Print and shaded views of the part. All mm, measured from the part's lowest x, y and z. Give positions to 0.01 mm unless a question says otherwise; leave off trailing zeros. Loops run counter-clockwise (first coordinate to the right, second up) from the corner with the lowest first, then second, coordinate; pieces in that order, holes last. Notation, with made-up numbers: M 3.25,4.5 L 55.25,4.5 A14 cw 55.25,10.5 Z; hole C 70,4 d10. An arc over 180 degrees is marked long. Answer in a Markdown table with one row per item.
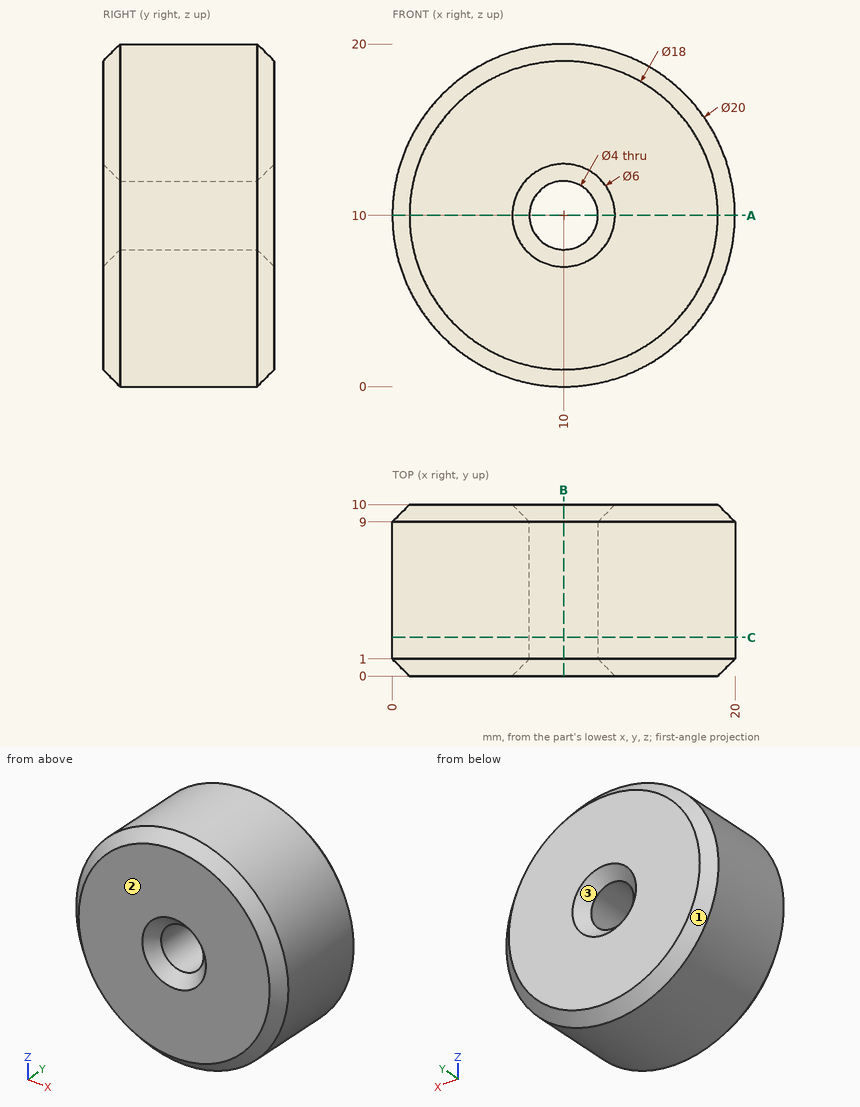
(1) Saw through at A-A, the plane z = 10. Give the cut face in (x, y).
Established:
| item | result |
|---|---|
| outline | M 0,1 L 1,0 L 7,0 L 8,1 L 8,9 L 7,10 L 1,10 L 0,9 Z; M 12,1 L 13,0 L 19,0 L 20,1 L 20,9 L 19,10 L 13,10 L 12,9 Z |
(2) Mould opens along X. For the marked faces 1, 2 and 3 say: pulls with the +X half, pulls with the -X half, needs draft (parallel to the pull), parting line crosses it, or undercut.
Established:
| item | result |
|---|---|
| face 1 | parting line crosses it |
| face 2 | needs draft |
| face 3 | undercut |
(3) Wall check: L1, parallel to Z at x = 10, y = 6.25; L2, parallel to X at y = 6.5, z = 9.75; L3, parallel to Z at x = 9.25, y = 4.5. Give the ranges that are in metal, low to high.
Established:
| item | result |
|---|---|
| L1 | z = 0 to 8, 12 to 20 |
| L2 | x = 0 to 8.02, 11.98 to 20 |
| L3 | z = 0.03 to 8.15, 11.85 to 19.97 |
(4) Flat gauge pins, fed straight in: P1, Ø1.5, axis at y = 2, z = 12.5, coming from the +X side; P2, Ø4, axis at x = 5.5, y = 8, coming from the +Z side; P3, Ø3, axis at y = 1.5, z = 4, coming from the +X side. Where does each tip first touch, or does it go through?
Established:
| item | result |
|---|---|
| P1 | stops at x = 19.85 |
| P2 | stops at z = 19.68 |
| P3 | stops at x = 18.93 |
(5) Saw through at C-C, the plane y = 2.25. Give the cut face in (x, z), and give its area (3 significant figures).
Established:
| item | result |
|---|---|
| outline | C 10,10 d20; hole C 10,10 d4 |
| area | 302 mm2 |
(6) Saw through at B-B, the plane x = 10. Give the cut face in (y, z), and give its area (3 significant figures).
Established:
| item | result |
|---|---|
| outline | M 0,1 L 1,0 L 9,0 L 10,1 L 10,7 L 9,8 L 1,8 L 0,7 Z; M 0,13 L 1,12 L 9,12 L 10,13 L 10,19 L 9,20 L 1,20 L 0,19 Z |
| area | 156 mm2 |
